For this review, take the finished solid that the model builds, in its own axes (mm). A direction names the side the tool comes from. Give positions to 0.01 mm unless a question says otherwise; leave off trailing zeros. Write each loop counter-clockwise with the first axis right and the second up, starting at its lowest first coordinate (ties: lowest second). Pieces come first, ordered by that corner, then holes. Notation, with made-up numbers: (43, 59) -> (80, 59) arc R18 cw to (80, 63) -> close; hole circle Ø5 at (36.5, 82). An arc over 180 degrees is marked (long way). Answer as CSV lines item,"result".
```python
from build123d import *

# Parameters (mm, degrees)
F3_DEPTH = 25
F5_DEPTH = 4


with BuildPart() as f1:
    # F0 (on Front) → F1 (revolve)
    with BuildSketch(Plane.XZ):
        with BuildLine():
            Line((4, 5), (4, 0))
            Line((4, 0), (15, 0))
            ThreePointArc((15, 0), (15.707107, 0.292893), (16, 1))
            Line((16, 1), (16, 1.456107))
            ThreePointArc((16, 1.456107), (15.622755, 2.625152), (14.633333, 3.35318))
            ThreePointArc((14.633333, 3.35318), (9.633139, 4.585612), (4.5, 5))
            Line((4.5, 5), (4, 5))
        make_face()
    revolve(axis=Axis((0, 0, 2.5), (0, 0, 1)))

    # F2 (on face) → F3 (cut)
    with BuildSketch(Plane.XY.offset(5)):
        with BuildLine():
            ThreePointArc((1.75, 10.5), (0, 12.25), (-1.75, 10.5))
            Line((-1.75, 10.5), (-1.75, 7.5))
            ThreePointArc((-1.75, 7.5), (0, 5.75), (1.75, 7.5))
            Line((1.75, 7.5), (1.75, 10.5))
        make_face()
        with BuildLine():
            Line((-7.5, 1.75), (-10.5, 1.75))
            ThreePointArc((-10.5, 1.75), (-12.25, 0), (-10.5, -1.75))
            Line((-10.5, -1.75), (-7.5, -1.75))
            ThreePointArc((-7.5, -1.75), (-5.75, 0), (-7.5, 1.75))
        make_face()
        with BuildLine():
            Line((-1.75, -7.5), (-1.75, -10.5))
            ThreePointArc((-1.75, -10.5), (0, -12.25), (1.75, -10.5))
            Line((1.75, -10.5), (1.75, -7.5))
            ThreePointArc((1.75, -7.5), (0, -5.75), (-1.75, -7.5))
        make_face()
        with BuildLine():
            Line((7.5, -1.75), (10.5, -1.75))
            ThreePointArc((10.5, -1.75), (12.25, 0), (10.5, 1.75))
            Line((10.5, 1.75), (7.5, 1.75))
            ThreePointArc((7.5, 1.75), (5.75, 0), (7.5, -1.75))
        make_face()
    extrude(amount=-F3_DEPTH, mode=Mode.SUBTRACT)

    # F4 (on face) → F5 (cut)
    with BuildSketch(Plane.XY.offset(5)):
        with BuildLine():
            Line((2.75, 2.75), (2.75, 10.5))
            ThreePointArc((2.75, 10.5), (0, 13.25), (-2.75, 10.5))
            Line((-2.75, 10.5), (-2.75, 2.75))
            Line((-2.75, 2.75), (-10.5, 2.75))
            ThreePointArc((-10.5, 2.75), (-13.25, 0), (-10.5, -2.75))
            Line((-10.5, -2.75), (-2.75, -2.75))
            Line((-2.75, -2.75), (-2.75, -10.5))
            ThreePointArc((-2.75, -10.5), (0, -13.25), (2.75, -10.5))
            Line((2.75, -10.5), (2.75, -2.75))
            Line((2.75, -2.75), (10.5, -2.75))
            ThreePointArc((10.5, -2.75), (13.25, 0), (10.5, 2.75))
            Line((10.5, 2.75), (2.75, 2.75))
        make_face()
    extrude(amount=-F5_DEPTH, mode=Mode.SUBTRACT)


solid = f1.part
```
Q1. For faces 5 (the flat face through (-3, -3, 0)), 6 (the flat face through (-2, -8, 1)), 7 (the cylindrical face through (12.25, -0.04, 0.51)), list the 3-axis set-ups (+Z, -Z, +X, -X, +Y, -Y) from which the entire face can be reached by the end or side of a thin tool; tool diameter is ignored.
Answer block:
face 5,"-Z, +X, -X, +Y, -Y"
face 6,"+Z"
face 7,"+Z, -Z"
Q2. Draft analysis for pull direction Y (two halves, no side actions). For faces 1 (the flat face through (-9, 1.75, 0.5)), 2 (the flat face through (-3, -3, 5)), 3 (the cylindrical face through (-3.47, -15.62, 1.23)), 4 (the flat face through (1.75, 9, 0.5)), state which applies: released by +Y, released by -Y, zero draft, split by the parting line, or undercut.
Answer block:
face 1,"undercut"
face 2,"zero draft"
face 3,"split by the parting line"
face 4,"undercut"
Q3. Clearance check with flat-ended pins moving along their axes: pin 1 (6.5 mm diameter, centred on x = 0, y = 0, fed in from +Z); pin 2 (10 mm diameter, centred on x = -3.5, y = 0.5, fed in from -Z); pin 3 (1.2 mm diameter, centred on y = -7, z = 3.5, fed in from -X); pin 4 (4.5 mm diameter, centred on x = 10, y = 1, fed in from +Z). State where each tip first meets the part, or that it passes through.
Answer block:
pin 1,"passes through"
pin 2,"stops at z = 0"
pin 3,"stops at x = -13.76"
pin 4,"stops at z = 4.68"
Q4. Add section A-A (z = 2.6). Write out the cut boundary in (x, y).
Answer block:
outline,"circle Ø31.28 at (0, 0); hole (-10.5, -2.75) -> (-2.9, -2.75) arc R4 ccw to (-2.75, -2.9) -> (-2.75, -10.5) arc R2.75 ccw to (2.75, -10.5) -> (2.75, -2.9) arc R4 ccw to (2.9, -2.75) -> (10.5, -2.75) arc R2.75 ccw to (10.5, 2.75) -> (2.9, 2.75) arc R4 ccw to (2.75, 2.9) -> (2.75, 10.5) arc R2.75 ccw to (-2.75, 10.5) -> (-2.75, 2.9) arc R4 ccw to (-2.9, 2.75) -> (-10.5, 2.75) arc R2.75 ccw to start"
Q5. To check wall thickness, follow probe 1 along Y at (x, z) = (0, 1.35); probe 2 along Z at (x, y) = (-11, 2.5); probe 3 along Y at (x, z) = (1.5, 2.2). State the ranges of each line that lie inside material, in increasing order. Write a range as [from, to].
Answer block:
probe 1,"y = [-16, -13.25], [13.25, 16]"
probe 2,"z = [0, 1]"
probe 3,"y = [-15.79, -12.8], [12.8, 15.79]"
Q6. Add section B-B (y = 0). State how many separate pieces and enclosed holes the cut face has, plus the area to 3 significant figures.
Answer block:
separate pieces,"4"
enclosed holes,"0"
area,"22.7 mm2"
